CAD build for the part. Positions are in the model's coordinates, mm. Coordinates: 2 decimals unless noted, no trailing zeros. Order: outer loops, then holes, each group sorted by start corner. A loop starts at its lowest first (then second) coordinate and runs counter-clockwise, first axis right, second up. Notation, with made-up numbers: (58.5, 42.5) - (113.5, 42.5) arc R32 ccw to (113.5, 80.5) - close; hole circle Ø10 at (-17, -3). An arc over 180 degrees is marked (long way). Return JSON: item names as keys, results as strings.
Autodesk Inventor part; units mm, degrees
ref_plane "YZ Plane" through (0, 0, 0) normal (1, 0, 0) x (0, 1, 0)
ref_plane "XZ Plane" through (0, 0, 0) normal (0, 1, 0) x (-1, 0, 0)
ref_plane "XY Plane" through (0, 0, 0) normal (0, 0, 1) x (1, 0, 0)
sketch "Sketch1" plane through (0, 0, 0) normal (0, 0, 1) x (1, 0, 0)
  circle A0 centre (0, 0) radius 7.5
  circle A1 centre (0, 0) radius 4
  dimension "d0" = 15
  dimension "d1" = 8
extrude "Extrusion1" add sketch "Sketch1" along normal blind 24
sketch "Sketch2" plane through (0, 0, 24) normal (0, 0, 1) x (1, 0, 0)
  arc A0 (0.5, 6) -> (-0.5, 6) centre (0, 6) ccw
  line L0 (-0.5, 6) -> (-0.5, 2.6094)
  line L1 (-0.5, 2.6094) -> (0.5, 2.6094)
  line L2 (0.5, 2.6094) -> (0.5, 6)
  line L3 (-4.5962, 3.8891) -> (-2.1987, 1.4916)
  arc A1 (-3.8891, 4.5962) -> (-4.5962, 3.8891) centre (-4.2426, 4.2426) ccw
  line L4 (-1.4916, 2.1987) -> (-3.8891, 4.5962)
  line L5 (-2.1987, 1.4916) -> (-1.4916, 2.1987)
  line L6 (-6, -0.5) -> (-2.6094, -0.5)
  arc A2 (-6, 0.5) -> (-6, -0.5) centre (-6, 0) ccw
  line L7 (-2.6094, 0.5) -> (-6, 0.5)
  line L8 (-2.6094, -0.5) -> (-2.6094, 0.5)
  line L9 (-3.8891, -4.5962) -> (-1.4916, -2.1987)
  arc A3 (-4.5962, -3.8891) -> (-3.8891, -4.5962) centre (-4.2426, -4.2426) ccw
  line L10 (-2.1987, -1.4916) -> (-4.5962, -3.8891)
  line L11 (-1.4916, -2.1987) -> (-2.1987, -1.4916)
  line L12 (0.5, -6) -> (0.5, -2.6094)
  arc A4 (-0.5, -6) -> (0.5, -6) centre (0, -6) ccw
  line L13 (-0.5, -2.6094) -> (-0.5, -6)
  line L14 (0.5, -2.6094) -> (-0.5, -2.6094)
  line L15 (4.5962, -3.8891) -> (2.1987, -1.4916)
  arc A5 (3.8891, -4.5962) -> (4.5962, -3.8891) centre (4.2426, -4.2426) ccw
  line L16 (1.4916, -2.1987) -> (3.8891, -4.5962)
  line L17 (2.1987, -1.4916) -> (1.4916, -2.1987)
  line L18 (6, 0.5) -> (2.6094, 0.5)
  arc A6 (6, -0.5) -> (6, 0.5) centre (6, 0) ccw
  line L19 (2.6094, -0.5) -> (6, -0.5)
  line L20 (2.6094, 0.5) -> (2.6094, -0.5)
  line L21 (3.8891, 4.5962) -> (1.4916, 2.1987)
  arc A7 (4.5962, 3.8891) -> (3.8891, 4.5962) centre (4.2426, 4.2426) ccw
  line L22 (2.1987, 1.4916) -> (4.5962, 3.8891)
  line L23 (1.4916, 2.1987) -> (2.1987, 1.4916)
  point P0 (0, 0)
  dimension "d4" = 1
  dimension "d7" = 360
extrude "Extrusion2" cut sketch "Sketch2" against normal blind 24
chamfer "Chamfer1" distance 0.635 angle 45 2 edges at (-7.5, 0, 24) (-7.5, 0, 0)
properties part number "Dry Bearing"
Item 1: Drop flat-ended pins along their axis: P1, Ø1.6, axis at x = 5.5, z = 16.5, coming from the +Y side; P2, Ø3, axis at y = -4.5, z = 9, coming from the -X side; P3, Ø0.6, axis at y = -5.5, z = 11, coming from the +X side. Give the stop position or say it passes through.
Findings below:
{"P1": "stops at y = 5.84", "P2": "stops at x = -6.87", "P3": "stops at x = 5.4"}
Item 2: Mould opens along Y. For faces 1 (the cylindrical face through (-7.493, -0.33, 11.841)), 2 (the cylindrical face through (-3.69, -1.54, 11.83)), 3 (the flat face through (4, -2, 0)) say: released by +Y, released by -Y, zero draft, split by the parting line, or undercut.
Findings below:
{"face 1": "split by the parting line", "face 2": "undercut", "face 3": "zero draft"}
Item 3: Wall check: L1, parallel to X at y = -4.25, z = 7.5; L2, parallel to Y at x = 4.5, z = 5.5; L3, parallel to Y at x = 4, z = 10.25. Give the ranges that are in metal, low to high. Write a range as [from, to].
Findings below:
{"L1": "x = [-6.18, -4.74], [-3.54, -0.5], [0.5, 3.54], [4.74, 6.18]", "L2": "y = [-6, -4.67], [-3.79, -0.5], [0.5, 3.79], [4.67, 6]", "L3": "y = [-6.34, -4.68], [-3.29, -0.5], [0.5, 3.29], [4.68, 6.34]"}
Item 4: Band-saw the part on A-A, the plane y = 0. List the corners of the cut face in (x, z) (3 decimals), then the cut area to 3 significant figures.
Findings below:
{"outline": "(-7.5, 0.635) - (-6.865, 0) - (-6.5, 0) - (-6.5, 24) - (-6.865, 24) - (-7.5, 23.365) - close; (6.5, 0) - (6.865, 0) - (7.5, 0.635) - (7.5, 23.365) - (6.865, 24) - (6.5, 24) - close", "area": "47.2 mm²"}
